Build history of the part. All positions in model axes, mm. Face numbers are marked on the shaded views. A direction names the side the tool comes from. Give positions to 0.01 mm unless a question says otherwise; leave off trailing zeros. Write each loop counter-clockwise with the first axis right and the second up, starting at its lowest first coordinate (ties: lowest second). Pieces come first, ordered by that corner, then holes.
Autodesk Inventor part; units mm, degrees
ref_plane "YZ Plane" through (0, 0, 0) normal (1, 0, 0) x (0, 1, 0)
ref_plane "XZ Plane" through (0, 0, 0) normal (0, 1, 0) x (-1, 0, 0)
ref_plane "XY Plane" through (0, 0, 0) normal (0, 0, 1) x (1, 0, 0)
sketch "Sketch1" plane through (0, 0, 0) normal (0, 1, 0) x (-1, 0, 0)
  arc A0 (-16.9706, -6) -> (-16.9706, 6) centre (0, 0) ccw
  circle A1 centre (0, 0) radius 32
  line L0 (-24, 0) -> (-24, 6)
  line L1 (-24, 0) -> (-24, -6)
  line L2 (-24, 6) -> (-16.9706, 6)
  line L3 (-24, -6) -> (-16.9706, -6)
  circle A2 centre (-100, 0) radius 12
  circle A3 centre (-100, 0) radius 21
  dimension "d0" = 36
  dimension "d1" = 64
  dimension "d3" = 6
  dimension "d4" = 6
  dimension "d6" = 24
  dimension "d7" = 42
extrude "Extrusion1" add sketch "Sketch1" along normal blind 36
sketch "Sketch2" plane through (100, 36, 0) normal (0, 1, 0) x (1, 0, 0)
  circle A0 centre (0, 0) radius 12
  circle A1 centre (0, 0) radius 21
  point P0 (-100, 0)
  dimension "d10" = 42
extrude "Extrusion2" cut sketch "Sketch2" against normal blind 12
sketch "Sketch3" plane through (0, 0, 0) normal (0, 1, 0) x (-1, 0, 0)
  circle A0 centre (-100, 0) radius 21
  line L0 (-100, -21) -> (-24.1454, -21)
  circle A1 centre (0, 0) radius 32
  line L1 (-100, 21) -> (-24.1454, 21)
  arc A2 (-100, -21) -> (-100, 21) centre (-100, 0) ccw
  circle A3 centre (0, 0) radius 30.971
  circle A4 centre (0, 0) radius 32
  circle A5 centre (-100, 0) radius 21
  dimension "d14" = 64
extrude "Extrusion3" add sketch "Sketch3" along normal blind 12 contours A0 L1 A1 L0
sketch "Sketch4" plane through (0, 12, 0) normal (0, 1, 0) x (1, 0, 0)
  arc A0 (24.1454, -21) -> (24.1454, 21) centre (0, 0) ccw
  line L0 (32, 0) -> (32, -6)
  line L1 (32, 0) -> (32, 6)
  arc A1 (100, 21) -> (100, -21) centre (100, 0) ccw
  line L2 (79, 0) -> (79, 6)
  line L3 (79, 0) -> (79, -6)
  line L4 (32, 6) -> (79, 6)
  line L5 (32, -6) -> (79, -6)
  dimension "d17" = 6
  dimension "d18" = 6
  dimension "d19" = 6
  dimension "d20" = 6
extrude "Extrusion4" add sketch "Sketch4" along normal blind 24.25
sketch "Sketch5" plane through (79, 12, -6) normal (0, 0, -1) x (-1, 0, 0)
  line L0 (0, 0) -> (0, 24.25)
  line L1 (0, 0) -> (47, 24.25)
  line L2 (47, 24.25) -> (0, 24.25)
  line L3 (0, 0) -> (-21, 0)
  line L4 (0, 24.25) -> (0, 0)
  point P0 (79, -12)
extrude "Extrusion5" cut sketch "Sketch5" against normal blind 24.25
properties part number "6 -  Part 4"
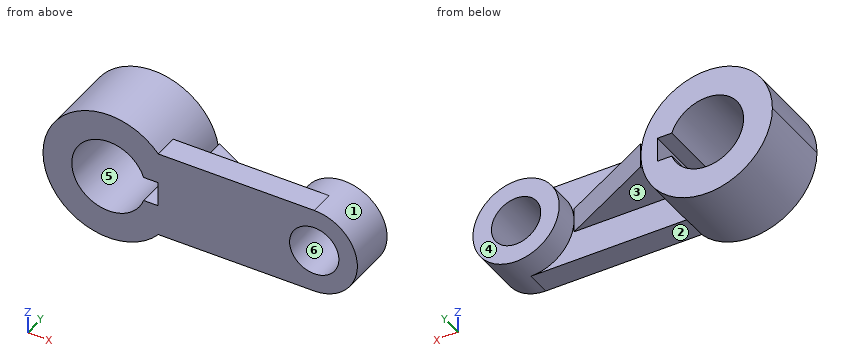
(1) Probe line 1 (X direction, y = 11.25, z = 0); line 2 (Z direction, x = 100, y = 8); line 3 (Z direction, x = 0, y = 18.5). List the from-to ranges inside material, lowest first.
(2) Mould opens along X. For the marked faces 4, 5 and 6 say: +X half, -X half, draft (parallel to the pull), parting line (faces both ways), or undercut.
(3) 3-axis set-ups, long thin cutter, end or side, ignore diameter. For the marked faces 1, 2 and 3: which of +Z, -Z, +X, -X, +Y, -Y reach the whole face in a straight line?
(4) Saw through at A-A, the plane x = 0. List the corners of the cut face in (y, z), plus the area to 3 significant figures.
(5) Drop flat-ended pins along their axis: pin 1 (13 mm diameter, centred on x = 53.5, y = 6, fed in from +Z); pin 2 (23 mm diameter, centred on x = 56.5, z = 7, fed in from +Y); pin 3 (3 mm diameter, centred on x = 69, z = 2, fed in from -Y); pin 4 (2 mm diameter, centred on y = 20, z = -2.5, fed in from +X). Give the stop position or say it passes through.
(6) Saw through at C-C, the plane y = 7.5. List the corners of the cut face in (x, z), plus the area to 3 significant figures.
Computed values:
1. line 1: x = -32 to -18, 24 to 88, 112 to 121
1. line 2: z = -21 to -12, 12 to 21
1. line 3: z = -32 to -18, 18 to 32
2. face 4: draft
2. face 5: undercut
2. face 6: undercut
3. face 1: +Y
3. face 2: -Z, +X, +Y, -Y
3. face 3: -Z, +Y
4. outline: (0, -32) - (36, -32) - (36, -18) - (0, -18) - close; (0, 18) - (36, 18) - (36, 32) - (0, 32) - close
4. area: 1,010 mm2
5. pin 1: stops at z = 21
5. pin 2: stops at y = 29.52
5. pin 3: stops at y = 0
5. pin 4: stops at x = 120.95
6. outline: (24.15, -21) - (100, -21) arc R21 ccw to (100, 21) - (24.15, 21) arc R32 ccw (long way) to start; hole (16.97, -6) - (24, -6) - (24, 6) - (16.97, 6) arc R18 ccw (long way) to start; hole circle Ø24 at (100, 0)
6. area: 5,320 mm2
